from build123d import *

# Parameters (mm, degrees)
ESQUISSE1_W        = 423
ESQUISSE1_H        = 133
ESQUISSE1_R        = 2.25
ESQUISSE1_R_2      = 1.5
ESQUISSE1_W_2      = 61
ESQUISSE1_H_2      = 29.5
ESQUISSE1_R_3      = 1.75
ESQUISSE1_R_4      = 2
BOSS_EXTRU_1_DEPTH = 1.2


with BuildPart() as part:
    # Esquisse1 → Boss.-Extru.1 (new body)
    with BuildSketch(Plane.XY):
        with Locations((-338.252753452, 101.126670585)):
            Rectangle(ESQUISSE1_W, ESQUISSE1_H)
        with Locations((-484.752753452, 69.626670585)):
            Circle(ESQUISSE1_R, mode=Mode.SUBTRACT)
        Polygon((-482.252753452, 112.126670585), (-482.252753452, 117.126670585), (-477.252753452, 117.126670585), (-477.252753452, 124.626670585), (-442.252753452, 124.626670585), (-442.252753452, 117.126670585), (-437.252753452, 117.126670585), (-437.252753452, 112.126670585), (-429.752753452, 112.126670585), (-429.752753452, 77.126670585), (-437.252753452, 77.126670585), (-437.252753452, 72.126670585), (-442.252753452, 72.126670585), (-442.252753452, 64.626670585), (-477.252753452, 64.626670585), (-477.252753452, 72.126670585), (-482.252753452, 72.126670585), (-482.252753452, 77.126670585), (-489.752753452, 77.126670585), (-489.752753452, 112.126670585), align=None, mode=Mode.SUBTRACT)
        with Locations((-434.752753452, 69.626670585)):
            Circle(ESQUISSE1_R, mode=Mode.SUBTRACT)
        with Locations((-349.252753452, 81.126670585)):
            Circle(ESQUISSE1_R_2, mode=Mode.SUBTRACT)
        with Locations((-349.252753452, 101.126670585)):
            Rectangle(ESQUISSE1_W_2, ESQUISSE1_H_2, mode=Mode.SUBTRACT)
        with Locations((-249.451641066, 45.126670585)):
            Circle(ESQUISSE1_R_3, mode=Mode.SUBTRACT)
        with Locations((-226.951641066, 45.126670585)):
            Circle(ESQUISSE1_R_3, mode=Mode.SUBTRACT)
        with Locations((-484.752753452, 119.626670585)):
            Circle(ESQUISSE1_R, mode=Mode.SUBTRACT)
        with Locations((-399.752753452, 101.126670585)):
            Circle(ESQUISSE1_R_4, mode=Mode.SUBTRACT)
        with Locations((-434.752753452, 119.626670585)):
            Circle(ESQUISSE1_R, mode=Mode.SUBTRACT)
        with Locations((-349.252753452, 121.126670585)):
            Circle(ESQUISSE1_R_2, mode=Mode.SUBTRACT)
        with Locations((-249.451641066, 157.126670585)):
            Circle(ESQUISSE1_R_3, mode=Mode.SUBTRACT)
        with Locations((-226.951641066, 157.126670585)):
            Circle(ESQUISSE1_R_3, mode=Mode.SUBTRACT)
    extrude(amount=BOSS_EXTRU_1_DEPTH)


solid = part.part
CAD build for the part. Positions are in the model's coordinates, mm. Give positions to 0.01 mm unless a question says otherwise; leave off trailing zeros. Write each loop counter-clockwise with the first axis right and the second up, starting at its lowest first coordinate (ties: lowest second). Pieces come first, ordered by that corner, then holes. Notation, with made-up numbers: (51, 19.5) - (97, 19.5) arc R24 cw to (97, 40.5) - close; hole circle Ø3 at (63, 52.25). An arc over 180 degrees is marked (long way). Answer as CSV lines item,"result".
Q1. Band-saw the part on B-B (z = 0.3). State how many separate pieces and enclosed holes the cut face has, and give its area (3 significant figures).
Result set:
separate pieces,"1"
enclosed holes,"13"
area,"51,300 mm²"
Q2. Band-saw the part on A-A (x = -472.5). Give the cut face in (y, z), and give its area (3 significant figures).
Result set:
outline,"(34.63, 0) - (64.63, 0) - (64.63, 1.2) - (34.63, 1.2) - close; (124.63, 0) - (167.63, 0) - (167.63, 1.2) - (124.63, 1.2) - close"
area,"87.6 mm²"
Q3. Drill centre lines: line 1 (X direction, y = 99, z = 0.5); line 2 (Y direction, x = -250, z = 1.1); line 3 (X direction, y = 70, z = 0.95). Where is each one in solid material? Low to high. Write a range as from..to.
Result set:
line 1,"-549.75..-489.75, -429.75..-379.75, -318.75..-126.75"
line 2,"34.63..43.46, 46.79..155.46, 158.79..167.63"
line 3,"-549.75..-486.97, -482.53..-477.25, -442.25..-436.97, -432.53..-126.75"
